```python
from build123d import *

# Parameters (mm, degrees)
SKETCH1_R             = 8.73125
BOSS_EXTRUDE1_DEPTH   = 116.84
SKETCH2_R             = 2.921
BOSS_EXTRUDE2_DEPTH   = 17.78
F_6_32_TAPPED_HOLE1_D = 2.7051
F_6_32_TAPPED_HOLE2_D = 2.7051
SKETCH4_R             = 1.8415
CUT_EXTRUDE1_DEPTH    = 137.028372284
SKETCH7_R             = 1.8415
CUT_EXTRUDE2_DEPTH    = 136.405147936


with BuildPart() as part:
    # Sketch1 → Boss-Extrude1 (new body)
    with BuildSketch(Plane.XY):
        with Locations(Location((0, 0, 0), (0, 0, 180))):
            Circle(SKETCH1_R)
    extrude(amount=BOSS_EXTRUDE1_DEPTH)

    # Sketch2 → Boss-Extrude2 (add)
    with BuildSketch(Plane.XY.offset(116.84)):
        Circle(SKETCH2_R)
    extrude(amount=BOSS_EXTRUDE2_DEPTH)

    # #6-32 Tapped Hole1 (through all)
    with Locations(Plane(origin=(0, 8.73125, 0), x_dir=(1, 0, 0), z_dir=(0, 1, 0))):
        with Locations((0, -62.23), (0, -95.25)):
            Hole(F_6_32_TAPPED_HOLE1_D / 2)

    # #6-32 Tapped Hole2 (through all)
    with Locations(Plane(origin=(2.921, 0, 0), x_dir=(0, 0, -1), z_dir=(1, 0, 0))):
        with Locations((-125.73, 0)):
            Hole(F_6_32_TAPPED_HOLE2_D / 2)

    # Sketch4 → Cut-Extrude1 (cut, through all)
    with BuildSketch(Plane(origin=(0, 8.73125, 0), x_dir=(1, 0, 0), z_dir=(0, 1, 0))):
        with Locations(Location((0, -62.23, 0), (0, 0, 270))):
            Circle(SKETCH4_R)
        with Locations(Location((0, -95.25, 0), (0, 0, 270))):
            Circle(SKETCH4_R)
    extrude(amount=-CUT_EXTRUDE1_DEPTH, mode=Mode.SUBTRACT)

    # Sketch7 → Cut-Extrude2 (cut, through all)
    with BuildSketch(Plane(origin=(2.921, 0, 0), x_dir=(0, 0, -1), z_dir=(1, 0, 0))):
        with Locations(Location((-125.73, 0, 0), (0, 0, 180))):
            Circle(SKETCH7_R)
    extrude(amount=-CUT_EXTRUDE2_DEPTH, mode=Mode.SUBTRACT)


solid = part.part
```
Part model, mm, in its own coordinate system. A direction names the side the tool comes from. Coordinates: 2 decimals unless noted, no trailing zeros. Order: outer loops, then holes, each group sorted by start corner. A loop starts at its lowest first (then second) coordinate and runs counter-clockwise, first axis right, second up. Notation, with made-up numbers: (11.25, -23) - (33.25, -23) arc R21 ccw to (33.25, 14) - close; hole circle Ø9 at (-2.5, -12.75). An arc over 180 degrees is marked (long way). Return JSON: item names as keys, results as strings. Group by question number.
Item 1: Pull direction X, two halves, no side cores. Call faces 3 (the face through (1.893, 8.524, 57.602)), 4 (the face through (0.04, -0.08, 123.89)), 5 (the face through (-0.71, 0.12, 63.93)), 6 (the face through (-1.634, 0.12, 96.1)): pulls with the +X half, pulls with the -X half, needs draft (parallel to the pull), parting line crosses it, or undercut.
Item 2: Which spindle directions (+Z, -Z, +X, -X, +Y, -Y) get a long thin tool onto all of the face, cutting with end or side? Do faces 1 (the face through (-0.38, 2.896, 125.606)), 2 (the face through (0, 0, 134.62)). Say none if no direction does.
Item 3: Cut at B-B (y = 0). List the corners of the cut face in (x, z).
Item 4: Cut at D-D (y = 6.75). List the corners of the cut face in (x, z), plus the area to 3 significant figures.
Item 5: Pin check, flat tips, straight feed: pin 1 (5 mm diameter, centred on x = -5.5, z = 97, fed in from -Y); pin 2 (10 mm diameter, centred on x = -6, z = 88, fed in from +Y); pin 3 (2 mm diameter, centred on y = -3, z = 115.5, fed in from +X). Stop position of each tip, or through.
Item 6: Cut at C-C (z = 62.23). List the corners of the cut face in (x, y), plus the area to 3 significant figures.
Item 7: Cut at A-A (x = 0). List the corners of the cut face in (y, z), plus the area to 3 significant figures.
Item 8: Drill centre lines: probe 1 along Z at (x, y) = (0, 2.5); probe 2 along Z at (x, y) = (0, -0.5); probe 3 along Z at (x, y) = (0, 0.75). Where is each one in solid material? Low to high. Write a range as from..to.
Check values:
{
 "1": {"face 3": "parting line crosses it", "face 4": "needs draft", "face 5": "undercut", "face 6": "undercut"},
 "2": {"face 1": "+Z", "face 2": "+Z, +X, -X, +Y, -Y"},
 "3": {"outline": "(-8.73, 0) - (8.73, 0) - (8.73, 116.84) - (2.92, 116.84) - (2.92, 123.89) - (-2.92, 123.89) - (-2.92, 116.84) - (-8.73, 116.84) - close; (-2.92, 127.57) - (2.92, 127.57) - (2.92, 134.62) - (-2.92, 134.62) - close; hole circle Ø3.68 at (0, 62.23); hole circle Ø3.68 at (0, 95.25)"},
 "4": {"outline": "(-5.54, 0) - (5.54, 0) - (5.54, 116.84) - (-5.54, 116.84) - close; hole circle Ø3.68 at (0, 62.23); hole circle Ø3.68 at (0, 95.25)", "area": "1,270 mm2"},
 "5": {"pin 1": "stops at y = -8.2", "pin 2": "stops at y = 8.67", "pin 3": "stops at x = 8.5"},
 "6": {"outline": "(-1.84, -8.53) - (-1.84, 8.53) arc R8.73 ccw to start; (1.84, -8.53) arc R8.73 ccw to (1.84, 8.53) - close", "area": "176 mm2"},
 "7": {"outline": "(-8.73, 0) - (8.73, 0) - (8.73, 60.39) - (-8.73, 60.39) - close; (-8.73, 64.07) - (8.73, 64.07) - (8.73, 93.41) - (-8.73, 93.41) - close; (-8.73, 97.09) - (8.73, 97.09) - (8.73, 116.84) - (2.92, 116.84) - (2.92, 134.62) - (-2.92, 134.62) - (-2.92, 116.84) - (-8.73, 116.84) - close; hole circle Ø3.68 at (0, 125.73)", "area": "2,000 mm2"},
 "8": {"probe 1": "z = 0..60.39, 64.07..93.41, 97.09..134.62", "probe 2": "z = 0..60.39, 64.07..93.41, 97.09..123.96, 127.5..134.62", "probe 3": "z = 0..60.39, 64.07..93.41, 97.09..124.05, 127.41..134.62"}
}
